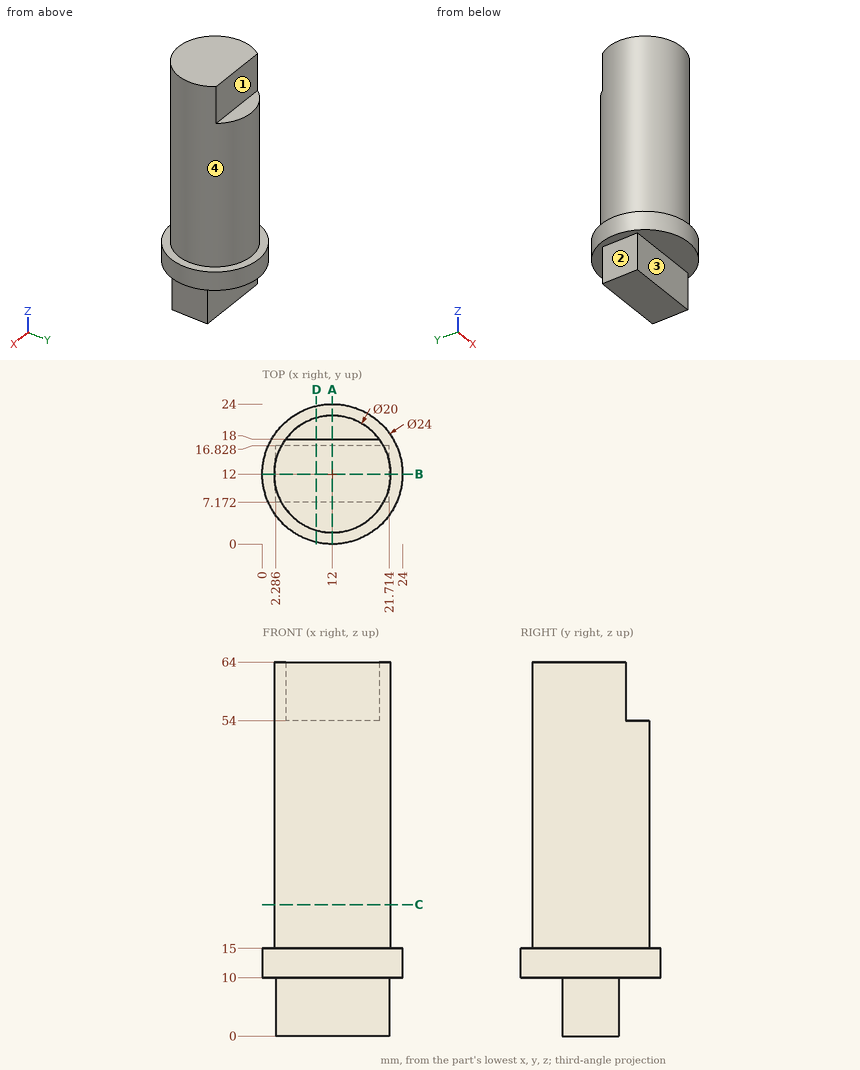
Here's the drawing with two shaded views (mm, measured from the low corner). I have some questions. A direction names the side the tool comes from. Give positions to 0.01 mm unless a question says otherwise; leave off trailing zeros. Order: outer loops, then holes, each group sorted by start corner. A loop starts at its lowest first (then second) coordinate and runs counter-clockwise, first axis right, second up. Notation, with made-up numbers: (60, 84.5) -> (71, 84.5) arc R22 cw to (71, 114.5) -> close; hole circle Ø4 at (-7.75, 7.25). An arc over 180 degrees is marked (long way). One line per item, written item: value. Start each with the question number.
1. Will these pins go through, and if not, where does the flat tip stop? pin 1 Ø3 at (x, z) = (8, 5.5) entering from +Y; pin 2 Ø1.2 at (x, y) = (8.5, 19) entering from +Z; pin 3 Ø5 at (x, z) = (11, 59) entering from +Y; pin 4 Ø12 at (x, y) = (14.5, 20.5) entering from -Z.
2. Imagine slicing it at B-B, the plane y = 12. List the corners of the cut face in (x, z) for me, plus the area to 3 significant figures.
3. Imagine slicing it at A-A, the plane x = 12. List the corners of the cut face in (y, z) for me, plus the area to 3 significant figures.
4. Imagine slicing it at D-D, the plane x = 9.25. List the corners of the cut face in (y, z) for me (1 decimal), plus the area to 3 significant figures.
5. For the marked faces 1, 2, 3 and 4, which set-ups out of +Z, -Z, +X, -X, +Y, -Y let a thin tool reach every point of the face, with its end or its side?
6. I need wall thicknesses on probe 1 along Z at (x, y) = (19.5, 18.5); probe 2 along Y at (x, z) = (10.25, 9.5); probe 3 along X at (y, z) = (16.75, 5). Which ranges of each line are inside material? Lowest first, please. Write a range as from..to.
7. Imagine slicing it at C-C, the plane z = 22.5. List the corners of the cut face in (x, y) for me.
Values follow:
1. pin 1: stops at y = 16.83
1. pin 2: stops at z = 54
1. pin 3: stops at y = 18
1. pin 4: stops at z = 0
2. outline: (0, 10) -> (2.29, 10) -> (2.29, 0) -> (21.71, 0) -> (21.71, 10) -> (24, 10) -> (24, 15) -> (22, 15) -> (22, 64) -> (2, 64) -> (2, 15) -> (0, 15) -> close
2. area: 1,290 mm2
3. outline: (0, 10) -> (7.17, 10) -> (7.17, 0) -> (16.83, 0) -> (16.83, 10) -> (24, 10) -> (24, 15) -> (22, 15) -> (22, 54) -> (18, 54) -> (18, 64) -> (2, 64) -> (2, 15) -> (0, 15) -> close
3. area: 1,160 mm2
4. outline: (0.3, 10) -> (7.2, 10) -> (7.2, 0) -> (16.8, 0) -> (16.8, 10) -> (23.7, 10) -> (23.7, 15) -> (21.6, 15) -> (21.6, 54) -> (18, 54) -> (18, 64) -> (2.4, 64) -> (2.4, 15) -> (0.3, 15) -> close
4. area: 1,120 mm2
5. face 1: +Z, +X, -X, +Y
5. face 2: -Z, -X, +Y, -Y
5. face 3: -Z, +X, -X, -Y
5. face 4: +Z
6. probe 1: z = 10..54
6. probe 2: y = 7.17..16.83
6. probe 3: x = 2.29..21.71
7. outline: circle Ø20 at (12, 12)
